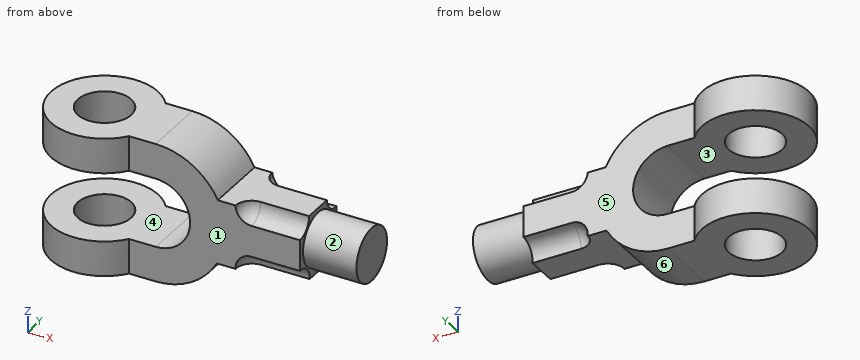
```python
from build123d import *

# Parameters (mm, degrees)
SKETCH1_W           = 20
SKETCH1_H           = 10
SKETCH1_8_R         = 10
BOSS_EXTRUDE4_DEPTH = 26
SKETCH4_W           = 46
SKETCH4_H           = 25.802584996
CUT_EXTRUDE2_DEPTH  = 26
SKETCH5_W           = 14.33272529
SKETCH5_H           = 12
CUT_EXTRUDE3_DEPTH  = 10
SKETCH6_W           = 18
SKETCH6_H           = 6
SKETCH7_R           = 6
CUT_EXTRUDE4_DEPTH  = 10
CIRPATTERN2_COUNT   = 4
CIRPATTERN3_COUNT   = 4


with BuildPart() as part:
    # Sketch1 → Revolve1 (revolve)
    with BuildSketch(Plane.XY, mode=Mode.PRIVATE) as revolve1_sk:
        with Locations((90, 5)):
            Rectangle(SKETCH1_W, SKETCH1_H)
    revolve(revolve1_sk.sketch.rotate(Axis((80, 0, 0), (1, 0, 0)), 180), axis=Axis((80, 0, 0), (1, 0, 0)))

    # Sketch1_8 → Boss-Extrude4 (add, symmetric)
    # profile 1 of 2: a face of its own
    with BuildSketch(Plane.XY):
        with BuildLine():
            Line((52, 12), (16, 12))
            ThreePointArc((16, 12), (-20, 0), (16, -12))
            Line((16, -12), (52, -12))
            Line((52, -12), (52, 12))
        make_face()
        with Locations(Location((0, 0, 0), (0, 0, 180))):
            Circle(SKETCH1_8_R, mode=Mode.SUBTRACT)
    # profile 2 of 2: a face of its own
    with BuildSketch(Plane.XY):
        Polygon((80, 12), (52, 12), (52, -12), (80, -12), (80, 0), (80, 10), align=None)
    extrude(amount=BOSS_EXTRUDE4_DEPTH, both=True)

    # Sketch4 → Cut-Extrude2 (cut, symmetric)
    with BuildSketch(Plane(origin=(0, 0, 0), x_dir=(1, 0, 0), z_dir=(0, 1, 0))):
        with Locations((3, 0)):
            Rectangle(SKETCH4_W, SKETCH4_H)
        with BuildLine():
            ThreePointArc((26, -12.901292498), (38.901292498, 0), (26, 12.901292498))
            Line((26, 12.901292498), (26, -12.901292498))
        make_face()
        with BuildLine():
            Line((48.864488658, 12.378011085), (80, 12.378011085))
            Line((80, 12.378011085), (80, 26))
            Line((80, 26), (26, 26))
            ThreePointArc((26, 26), (39.307360966, 22.336386102), (48.864488658, 12.378011085))
        make_face()
        with BuildLine():
            Line((26, -26), (80, -26))
            Line((80, -26), (79.906653098, -11.621988915))
            Line((79.906653098, -11.621988915), (49.257888418, -11.621988915))
            ThreePointArc((49.257888418, -11.621988915), (39.671654768, -22.115285571), (26, -26))
        make_face()
    extrude(amount=CUT_EXTRUDE2_DEPTH, both=True, mode=Mode.SUBTRACT)

    # Sketch5 → Cut-Extrude3 (cut)
    with BuildSketch(Plane(origin=(80, 0, 0), x_dir=(0, 0, -1), z_dir=(1, 0, 0))):
        with Locations((-18.833637355, 6)):
            Rectangle(SKETCH5_W, SKETCH5_H)
        with Locations((-18.833637355, -6)):
            Rectangle(SKETCH5_W, SKETCH5_H)
    extrude(amount=-CUT_EXTRUDE3_DEPTH, mode=Mode.SUBTRACT)

    # Sketch6 → Cut-Revolve3 (revolve, cut)
    with BuildSketch(Plane.XY.offset(11.621988915)):
        with Locations((70.906653098, -9)):
            Rectangle(SKETCH6_W, SKETCH6_H)
        with BuildLine():
            Line((55.906653098, -12), (61.906653098, -12))
            Line((61.906653098, -12), (61.906653098, -6))
            ThreePointArc((61.906653098, -6), (57.664012411, -7.757359313), (55.906653098, -12))
        make_face()
    cut_revolve3 = revolve(axis=Axis((81.079011265, -12, 11.621988915), (-1, 0, 0)), mode=Mode.SUBTRACT)

    # Sketch7 → Cut-Extrude4 (cut)
    with BuildSketch(Plane.ZY.offset(-79.906653098)):
        with Locations((11.621988915, -12)):
            Circle(SKETCH7_R)
    cut_extrude4 = extrude(amount=-CUT_EXTRUDE4_DEPTH, mode=Mode.SUBTRACT)

    # CirPattern2: Cut-Revolve3 ×4 about axis
    cirpattern2_axis = Axis((81.079011265, -12, 11.621988915), (1, 0, 0))
    for i in range(1, CIRPATTERN2_COUNT):
        add(cut_revolve3.rotate(cirpattern2_axis, i * 360 / CIRPATTERN2_COUNT), mode=Mode.SUBTRACT)

    # CirPattern3: Cut-Revolve3, Cut-Extrude4 ×4 about axis
    cirpattern3_axis = Axis((0, 0, 0), (1, 0, 0))
    add([cut_revolve3.rotate(cirpattern3_axis, i * 360 / CIRPATTERN3_COUNT) for i in range(1, CIRPATTERN3_COUNT)], mode=Mode.SUBTRACT)
    add([cut_extrude4.rotate(cirpattern3_axis, i * 360 / CIRPATTERN3_COUNT) for i in range(1, CIRPATTERN3_COUNT)], mode=Mode.SUBTRACT)


solid = part.part
```
Could you check a few things on this model? Use its own coordinates, in mm. Face numbers are marked on the shaded views. A direction names the side the tool comes from. Coordinates: 2 decimals unless noted, no trailing zeros. Loops run counter-clockwise (first coordinate to the right, second up) from the corner with the lowest first, then second, coordinate; pieces in that order, holes last.
1) Imagine slicing it at C-C (z = 0). List the corners of the cut face in (x, y) for me, and give its area (3 significant figures).
Reported:
outline: (38.9, -12) - (80, -12) - (80, -10) - (100, -10) - (100, 10) - (80, 10) - (80, 12) - (38.9, 12) - close
area: 1,390 mm2
2) Please list where these lines run through material, in increasing order: line 1 along Z through (x, y) = (-11, 12); line 2 along Y through (x, z) = (0, 20); line 3 along Y through (x, z) = (-6.5, 23).
Reported:
line 1: z = -26 to -12.9, 12.9 to 26
line 2: y = -20 to -10, 10 to 20
line 3: y = -18.91 to -7.6, 7.6 to 18.91
3) Imagine slicing it at A-A (y = 0). List the corners of the cut face in (x, z) for me, and give its area (3 significant figures).
Reported:
outline: (-20, -26) - (-10, -26) - (-10, -12.9) - (-20, -12.9) - close; (-20, 12.9) - (-10, 12.9) - (-10, 26) - (-20, 26) - close; (10, -26) - (26, -26) arc R26 ccw to (48.86, -12.38) - (80, -12.38) - (80, -10) - (100, -10) - (100, 10) - (80, 10) - (80, 11.67) - (79.91, 11.67) - (79.91, 11.62) - (49.26, 11.62) arc R26 ccw to (26, 26) - (10, 26) - (10, 12.9) - (26, 12.9) arc R12.9 cw to (26, -12.9) - (10, -12.9) - close
area: 2,580 mm2
4) Which directions (+Z, -Z, +X, -X, +Y, -Y) give clear straight access to the entire face, cutting with the end or side of a thin tool? Please do the marked faces 1 and 2.
Reported:
face 1: +Z, -Z, +X, -Y
face 2: +X
5) Will these pins go through, and if not, where does the flat tip stop? pin 1 Ø19 at (x, y) = (62.5, -1.5) entering from +Z; pin 2 Ø12 at (y, z) = (12, -18.5) entering from -X; pin 3 Ø12 at (x, z) = (7, 9) entering from -Y.
Reported:
pin 1: stops at z = 11.62
pin 2: stops at x = -19.08
pin 3: stops at y = -19.85
6) Imagine slicing it at B-B (x = 23). List the corners of the cut face in (y, z) for me.
Reported:
outline: (-12, -26) - (12, -26) - (12, -12.9) - (-12, -12.9) - close; (-12, 12.9) - (12, 12.9) - (12, 26) - (-12, 26) - close
7) Imagine slicing it at D-D (x = 0). List the corners of the cut face in (y, z) for me, and give its area (3 significant figures).
Reported:
outline: (-20, -26) - (-10, -26) - (-10, -12.9) - (-20, -12.9) - close; (-20, 12.9) - (-10, 12.9) - (-10, 26) - (-20, 26) - close; (10, -26) - (20, -26) - (20, -12.9) - (10, -12.9) - close; (10, 12.9) - (20, 12.9) - (20, 26) - (10, 26) - close
area: 524 mm2
8) Thinking about a two-plate mould opening in Z: for the marked faces 3, 4, 5 and 6, which applies, released by +Z, released by -Z, zero draft, split by the parting line, or undercut?
Reported:
face 3: undercut
face 4: undercut
face 5: zero draft
face 6: released by -Z
